Check sheet for the modelled part. Datum: model origin and axes. Units: mm. Face numbers are marked on the shaded views. Coordinates: 2 decimals unless noted, no trailing zeros. Order: outer loops, then holes, each group sorted by start corner. A loop starts at its lowest first (then second) coordinate and runs counter-clockwise, first axis right, second up.
1. Draft check along X on the marked faces 1, 2, 3 and 4. Enter one of: released by +X, released by -X, zero draft, split by the parting line, or undercut.
2. Cross-section at A-A (y = 43). Enter the section's corners in (x, z).
3. Gauge pin test, flat end, axial feed: pin 1 Ø2.5 at (x, y) = (10, 23) entering from +Z. Record the tip position at first contact, or that the pin passes through.
4. Cross-section at B-B (x = 20). Enter the section's corners in (y, z), then the cut area to 3 significant figures.
5. Cross-section at C-C (x = 10). Enter the section's corners in (y, z), then the cut area to 3 significant figures.
6. Cross-section at D-D (z = 5.25). Enter the section's corners in (x, y).
7. Thickness scan on line 1 (Y direction, x = 10, z = 6.5); line 2 (Y direction, x = 20, z = 3.5); line 3 (Y direction, x = 30.5, z = 5). Record the ranges inside material, lowest first.
```python
from build123d import *

# Parameters (mm, degrees)
ESQUISSE1_W             = 40
ESQUISSE1_H             = 53
BOSS_EXTRU_1_DEPTH      = 9
ESQUISSE2_R             = 2
ESQUISSE2_R_2           = 3.4
ENL_V_MAT_EXTRU_1_DEPTH = 68.007462271
CONG_1_R                = 4


with BuildPart() as part:
    # Esquisse1 → Boss.-Extru.1 (new body)
    with BuildSketch(Plane.XY):
        with Locations((20, 26.5)):
            Rectangle(ESQUISSE1_W, ESQUISSE1_H)
    extrude(amount=BOSS_EXTRU_1_DEPTH)

    # Esquisse2 → Enlèv. mat.-Extru.1 (cut, through all)
    with BuildSketch(Plane.XY.offset(9)):
        with Locations((10, 43)):
            Circle(ESQUISSE2_R)
        with Locations(Location((30, 43, 0), (0, 0, 180))):
            Circle(ESQUISSE2_R)
        with Locations((30, 23)):
            Circle(ESQUISSE2_R)
        with Locations(Location((10, 23, 0), (0, 0, 180))):
            Circle(ESQUISSE2_R)
        with Locations((20, 9)):
            Circle(ESQUISSE2_R_2)
    extrude(amount=-ENL_V_MAT_EXTRU_1_DEPTH, mode=Mode.SUBTRACT)

    # Congé1
    cong_1_edges = [part.edges().sort_by_distance(p)[0] for p in [
        (0, 53, 4.5),
        (40, 53, 4.5),
        (40, 0, 4.5),
        (0, 0, 4.5),
    ]]
    fillet(cong_1_edges, radius=CONG_1_R)


solid = part.part
```
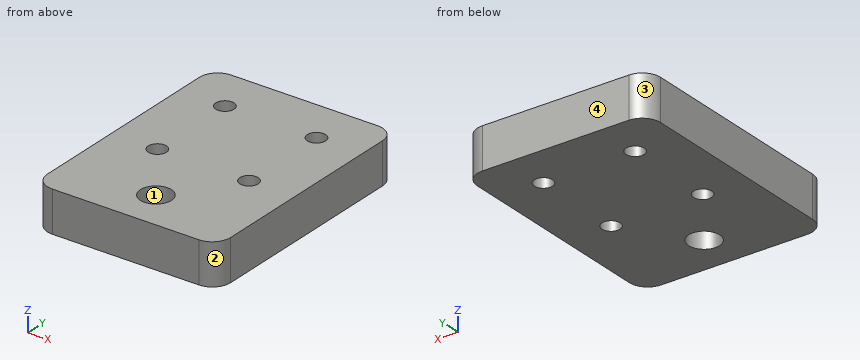
Data:
1. face 1: undercut
1. face 2: released by +X
1. face 3: released by -X
1. face 4: zero draft
2. outline: (0, 0) - (8, 0) - (8, 9) - (0, 9) - close; (12, 0) - (28, 0) - (28, 9) - (12, 9) - close; (32, 0) - (40, 0) - (40, 9) - (32, 9) - close
3. pin 1: passes through
4. outline: (0, 0) - (5.6, 0) - (5.6, 9) - (0, 9) - close; (12.4, 0) - (53, 0) - (53, 9) - (12.4, 9) - close
4. area: 416 mm2
5. outline: (0, 0) - (21, 0) - (21, 9) - (0, 9) - close; (25, 0) - (41, 0) - (41, 9) - (25, 9) - close; (45, 0) - (53, 0) - (53, 9) - (45, 9) - close
5. area: 405 mm2
6. outline: (0, 4) arc R4 ccw to (4, 0) - (36, 0) arc R4 ccw to (40, 4) - (40, 49) arc R4 ccw to (36, 53) - (4, 53) arc R4 ccw to (0, 49) - close; hole circle Ø4 at (10, 23); hole circle Ø4 at (10, 43); hole circle Ø6.8 at (20, 9); hole circle Ø4 at (30, 23); hole circle Ø4 at (30, 43)
7. line 1: y = 0 to 21, 25 to 41, 45 to 53
7. line 2: y = 0 to 5.6, 12.4 to 53
7. line 3: y = 0 to 21.06, 24.94 to 41.06, 44.94 to 53
